Job drawing, mm, ordinate dimensions from the low corner. One solid piece. A direction names the side the tool comes from. Coordinates: 2 decimals unless noted, no trailing zeros. Write each loop counter-clockwise with the first axis right and the second up, starting at its lowest first coordinate (ties: lowest second). Pieces come first, ordered by that corner, then holes. Notation, with made-up numbers: (68, -34) - (107, -34) arc R27 cw to (107, 1) - close; hole circle Ø8 at (48, 53.5). An arc over 180 degrees is marked (long way). Put each result on its own line as item: value. Start each with the question number.
1. Drop flat-ended pins along their axis: P1, Ø8, axis at y = 13, z = 35.5, coming from the +X side; P2, Ø10, axis at x = 21.5, z = 30, coming from the +Y side; P3, Ø1, axis at x = 41.5, y = 8.5, coming from the +Z side. Give the stop position or say it passes through.
2. Saw through at C-C, the plane x = 39.5. Write the cut outline in (y, z).
3. Which spindle directions (+Z, -Z, +X, -X, +Y, -Y) get a long thin tool onto all of the face, cutting with end or side? Do the marked faces 1, 2, 3, 4 and 5. Say none if no direction does.
4. Drill centre lines: L1, parallel to Y at x = 34, z = 5; L2, parallel to X at y = 38, z = 8; L3, parallel to Z at x = 25.5, y = 7. Where is each one in solid material? Low to high. Write a range as from..to.
5. Saw through at B-B, the plane y = 39. Write the cut outline in (x, z).
6. Saw through at A-A, the plane x = 25. Write the cut outline in (y, z), plus the area to 3 significant figures.
7. Saw through at D-D, the plane z = 13.5. Write the cut outline in (x, y).
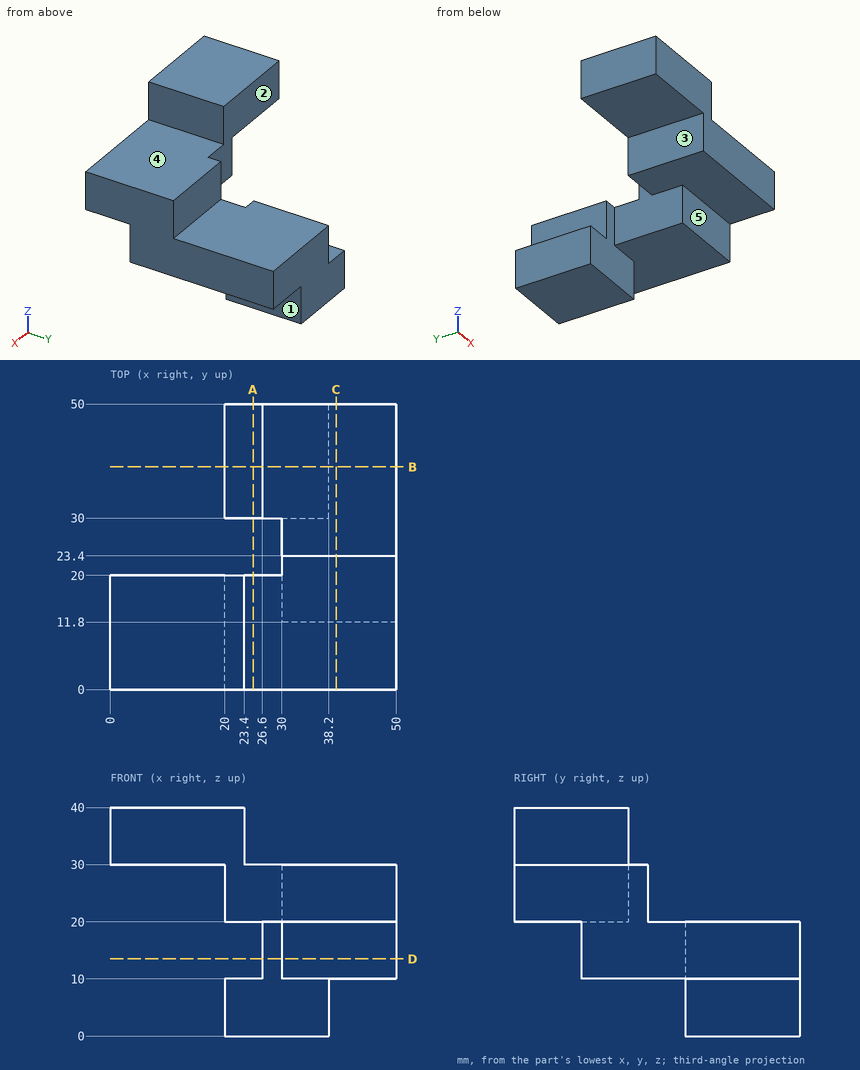
Final values:
1. P1: stops at x = 23.4
1. P2: stops at y = 20
1. P3: stops at z = 30
2. outline: (0, 20) - (11.8, 20) - (11.8, 10) - (50, 10) - (50, 20) - (23.4, 20) - (23.4, 30) - (0, 30) - close
3. face 1: -Z, +X, +Y, -Y
3. face 2: +Z, -Z, -X, +Y
3. face 3: -Z, -X, +Y, -Y
3. face 4: +Z, +X, +Y, -Y
3. face 5: -Z, +X, -X, -Y
4. L1: y = 30..50
4. L2: x = 20..38.2
4. L3: z = 20..30
5. outline: (20, 0) - (38.2, 0) - (38.2, 10) - (50, 10) - (50, 20) - (26.6, 20) - (26.6, 10) - (20, 10) - close
6. outline: (0, 20) - (20, 20) - (20, 30) - (0, 30) - close; (30, 0) - (50, 0) - (50, 10) - (30, 10) - close
6. area: 400 mm²
7. outline: (26.6, 30) - (30, 30) - (30, 11.8) - (50, 11.8) - (50, 50) - (26.6, 50) - close
